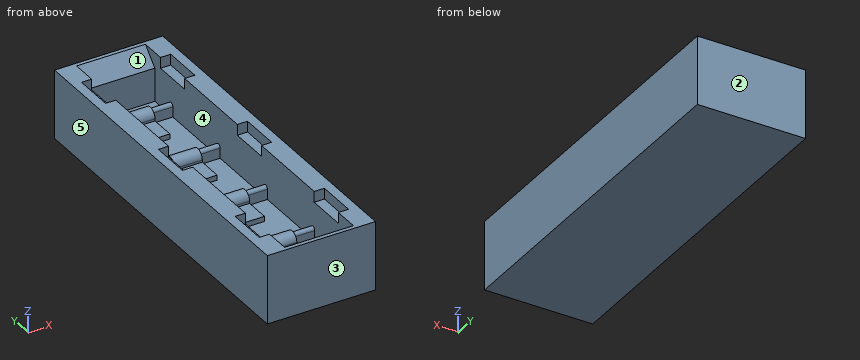
```python
from build123d import *

# Parameters (mm, degrees)
F0_W     = 22.225
F0_H     = 101.6
F1_DEPTH = 6.35
F3_DEPTH = 4.445
F5_DEPTH = 6.6675
F6_W     = 34.925
F6_H     = 114.3
F6_W_2   = 22.225
F6_H_2   = 101.6
F7_DEPTH = 22.225
F8_W     = 3.302
F8_H     = 12.954
F9_DEPTH = 3.5052
F10_SIZE = 5.08


with BuildPart() as f1:
    # F0 (on Top) → F1 (new body)
    with BuildSketch(Plane.XY):
        Rectangle(F0_W, F0_H)
    extrude(amount=-F1_DEPTH)

    # F2 (on Right) → F3 (join, symmetric)
    with BuildSketch(Plane.YZ):
        with BuildLine():
            Line((-44.577, 0), (-31.623, 0))
            Line((-31.623, 0), (-31.623, 2.3495))
            ThreePointArc((-31.623, 2.3495), (-34.0995, 4.826), (-36.576, 2.3495))
            Line((-36.576, 2.3495), (-36.576, 1.651))
            Line((-36.576, 1.651), (-44.577, 1.651))
            Line((-44.577, 1.651), (-44.577, 0))
        make_face()
        with BuildLine():
            Line((-19.177, 0), (-6.223, 0))
            Line((-6.223, 0), (-6.223, 2.3495))
            ThreePointArc((-6.223, 2.3495), (-8.6995, 4.826), (-11.176, 2.3495))
            Line((-11.176, 2.3495), (-11.176, 1.651))
            Line((-11.176, 1.651), (-19.177, 1.651))
            Line((-19.177, 1.651), (-19.177, 0))
        make_face()
        with BuildLine():
            Line((6.223, 0), (19.177, 0))
            Line((19.177, 0), (19.177, 2.3495))
            ThreePointArc((19.177, 2.3495), (16.7005, 4.826), (14.224, 2.3495))
            Line((14.224, 2.3495), (14.224, 1.651))
            Line((14.224, 1.651), (6.223, 1.651))
            Line((6.223, 1.651), (6.223, 0))
        make_face()
        with BuildLine():
            Line((31.623, 0), (44.577, 0))
            Line((44.577, 0), (44.577, 2.3495))
            ThreePointArc((44.577, 2.3495), (42.1005, 4.826), (39.624, 2.3495))
            Line((39.624, 2.3495), (39.624, 1.651))
            Line((39.624, 1.651), (31.623, 1.651))
            Line((31.623, 1.651), (31.623, 0))
        make_face()
    extrude(amount=F3_DEPTH, both=True)

    # F4 (on face) → F5 (join, through all)
    with BuildSketch(Plane.YZ.offset(4.445)):
        with BuildLine():
            ThreePointArc((-33.147, 3.302), (-34.0995, 4.2545), (-35.052, 3.302))
            Line((-35.052, 3.302), (-35.052, 0))
            Line((-35.052, 0), (-33.147, 0))
            Line((-33.147, 0), (-33.147, 3.302))
        make_face()
        with BuildLine():
            Line((-9.652, 3.302), (-9.652, 0))
            Line((-9.652, 0), (-7.747, 0))
            Line((-7.747, 0), (-7.747, 3.302))
            ThreePointArc((-7.747, 3.302), (-8.6995, 4.2545), (-9.652, 3.302))
        make_face()
        with BuildLine():
            Line((15.748, 3.302), (15.748, 0))
            Line((15.748, 0), (17.653, 0))
            Line((17.653, 0), (17.653, 3.302))
            ThreePointArc((17.653, 3.302), (16.7005, 4.2545), (15.748, 3.302))
        make_face()
        with BuildLine():
            Line((41.148, 3.302), (41.148, 0))
            Line((41.148, 0), (43.053, 0))
            Line((43.053, 0), (43.053, 3.302))
            ThreePointArc((43.053, 3.302), (42.1005, 4.2545), (41.148, 3.302))
        make_face()
    extrude(amount=F5_DEPTH)

    # F6 (on face) → F7 (join)
    with BuildSketch(Plane(origin=(0, 0, -6.35), x_dir=(1, 0, 0), z_dir=(0, 0, -1))):
        Rectangle(F6_W, F6_H)
        Rectangle(F6_W_2, F6_H_2, mode=Mode.SUBTRACT)
    extrude(amount=-F7_DEPTH)

    # F8 (on face) → F9 (cut)
    with BuildSketch(Plane.XY.offset(15.875)):
        with Locations((-12.7635, 41.275)):
            Rectangle(F8_W, F8_H)
        with Locations((-12.7635, 0)):
            Rectangle(F8_W, F8_H)
        with Locations((-12.7635, -41.275)):
            Rectangle(F8_W, F8_H)
        with Locations((12.7635, 41.275)):
            Rectangle(F8_W, F8_H)
        with Locations((12.7635, 0)):
            Rectangle(F8_W, F8_H)
        with Locations((12.7635, -41.275)):
            Rectangle(F8_W, F8_H)
    extrude(amount=-F9_DEPTH, mode=Mode.SUBTRACT)

    # F10
    f10_edges = [f1.edges().sort_by_distance(p)[0] for p in [
        (0, 50.8, 15.875),
        (0, -50.8, 15.875),
    ]]
    chamfer(f10_edges, length=F10_SIZE)


solid = f1.part
```
Model file for the job. Use its own axes, mm. Face numbers are marked on the shaded views. A direction names the side the tool comes from. Round coordinates to 2 decimals unless told otherwise and drop trailing zeros. Order: outer loops, then holes, each group sorted by start corner. A loop starts at its lowest first (then second) coordinate and runs counter-clockwise, first axis right, second up. Notation, with made-up numbers: (64, -28) -> (111, -28) arc R35 cw to (111, 9) -> close; hole circle Ø6 at (26.5, 28.5). An arc over 180 degrees is marked (long way). Use one line per item in the form item = value.
Item 1: Drill centre lines: line 1 (Y direction, x = 10.5, z = 2); line 2 (X direction, y = -21.5, z = 3.5); line 3 (Z direction, x = -10, y = -27). Where is each one in solid material? Low to high.
Returned:
line_1 = -57.15 to -50.8, -35.05 to -33.15, -9.65 to -7.75, 15.75 to 17.65, 41.15 to 43.05, 50.8 to 57.15
line_2 = -17.46 to -11.11, 11.11 to 17.46
line_3 = -6.35 to 0
Item 2: Pull direction Y, two halves, no side cores. Call the marked faces 3, 4 and 5: released by +Y, released by -Y, zero draft, split by the parting line, or undercut.
Returned:
face_3 = released by -Y
face_4 = undercut
face_5 = zero draft
Item 3: Cut at B-B, the plane z = 6.5. Write the cut outline in (x, y).
Returned:
outline = (-17.46, -57.15) -> (17.46, -57.15) -> (17.46, 57.15) -> (-17.46, 57.15) -> close; hole (-11.11, -50.8) -> (11.11, -50.8) -> (11.11, 50.8) -> (-11.11, 50.8) -> close
Item 4: Tool access for the marked faces 1 and 2: list every direction of +Z, -Z, +X, -X, +Y, -Y with a clear straight run to the whole face (end or side of a thin tool).
Returned:
face_1 = +Z
face_2 = +Z, -Z, +X, -X, +Y
Item 5: Flat gauge pins, fed straight in: pin 1 Ø1 at (x, y) = (5, -13) entering from +Z; pin 2 Ø2.5 at (x, y) = (-12, -39) entering from +Z. Where does each tip first touch, or does it go through?
Returned:
pin_1 = 0
pin_2 = 12.37
